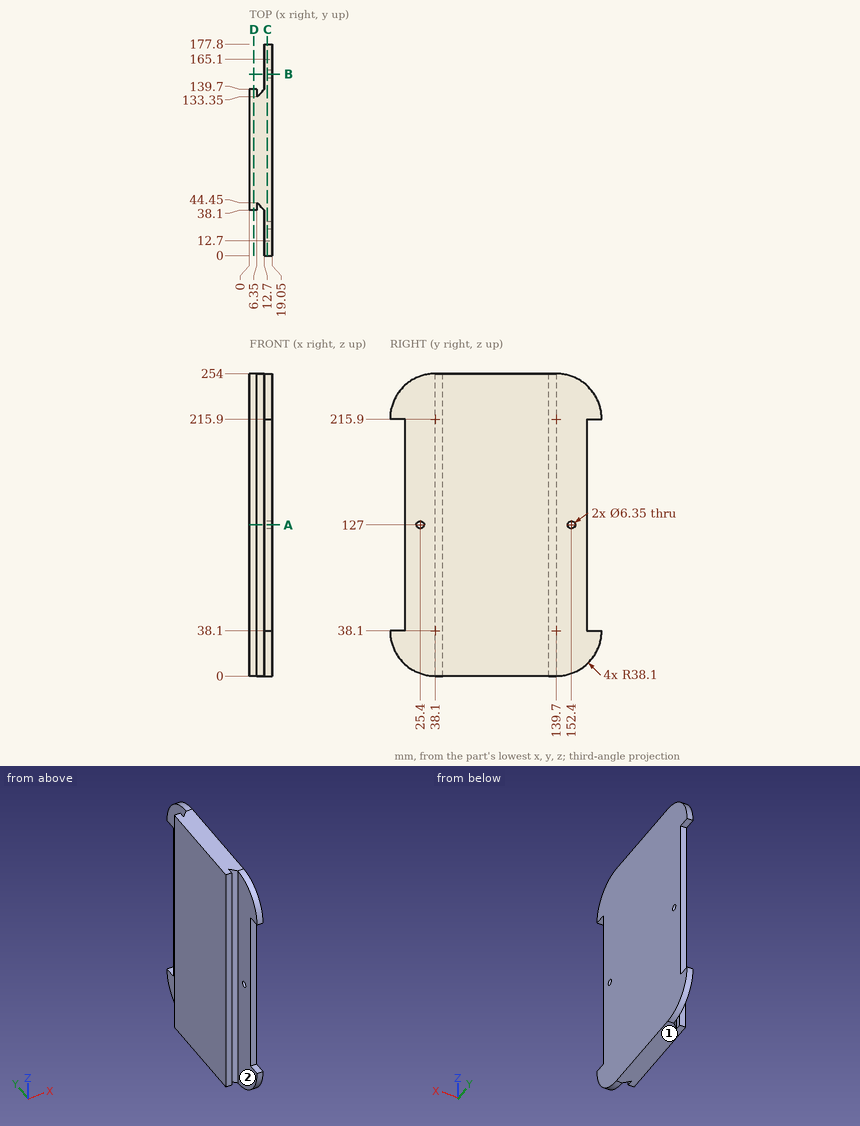
Here's the drawing with two shaded views (mm, measured from the low corner). I have some questions. A direction names the side the tool comes from. Round coordinates to 2 decimals unless told otherwise and drop trailing zeros. Loops run counter-clockwise (first coordinate to the right, second up) from the corner with the lowest first, then second, coordinate; pieces in that order, holes last.
Item 1: Suppose I cut it at C-C, the plane x = 15.25. Write out the boundary of the cut face in (y, z) (3 decimals).
Item 2: Suppose I cut it at B-B, the plane y = 152.4. Write out the boundary of the cut face in (x, z) (3 decimals), then the cut area to 3 significant figures.
Item 3: Suppose I cut it at D-D, the plane x = 3.75. Write out the boundary of the cut face in (y, z), then the cut area to 3 significant figures.
Item 4: Which directions (+Z, -Z, +X, -X, +Y, -Y) give clear straight access to the entire face, cutting with the end or side of a thin tool? Please do the marked faces 1 and 2.
Item 5: Suppose I cut it at A-A, the plane z = 127. Write out the boundary of the cut face in (x, y) (3 decimals).
Item 6: Will these pins go through, and if not, where does the flat tip stop? pin 1 Ø1.9 at (x, z) = (15.5, 133.5) entering from +Y; pin 2 Ø5 at (x, y) = (16.5, 174) entering from +Z (3 decimals); pin 3 Ø8.5 at (y, z) = (25.4, 127) entering from +X; pin 4 Ø3 at (x, z) = (1.5, 107) entering from -Y.
Item 7: Please list where these lines run through material, in increasing order: L1, parallel to Y at x = 14, z = 127 (3 decimals); L2, parallel to Y at x = 4.5, z = 175.5; L3, parallel to X at y = 150.5, z = 163.
Reported:
1. outline: (0, 38.1) arc R38.1 ccw to (38.1, 0) - (139.7, 0) arc R38.1 ccw to (177.8, 38.1) - (165.1, 38.1) - (165.1, 215.9) - (177.8, 215.9) arc R38.1 ccw to (139.7, 254) - (38.1, 254) arc R38.1 ccw to (0, 215.9) - (12.7, 215.9) - (12.7, 38.1) - close; hole circle Ø6.35 at (25.4, 127); hole circle Ø6.35 at (152.4, 127)
2. outline: (12.7, 2.179) - (19.05, 2.179) - (19.05, 123.825) - (12.7, 123.825) - close; (12.7, 130.175) - (19.05, 130.175) - (19.05, 251.821) - (12.7, 251.821) - close
2. area: 1,540 mm2
3. outline: (38.1, 0) - (139.7, 0) - (139.7, 254) - (38.1, 254) - close
3. area: 25,800 mm2
4. face 1: -Z, +X, -X, +Y, -Y
4. face 2: +Z, -Z, -X, -Y
5. outline: (0, 38.1) - (6.35, 38.1) - (6.35, 44.45) - (12.7, 38.1) - (12.7, 28.575) - (19.05, 28.575) - (19.05, 149.225) - (12.7, 149.225) - (12.7, 139.7) - (6.35, 133.35) - (6.35, 139.7) - (0, 139.7) - close; (12.7, 12.7) - (19.05, 12.7) - (19.05, 22.225) - (12.7, 22.225) - close; (12.7, 155.575) - (19.05, 155.575) - (19.05, 165.1) - (12.7, 165.1) - close
6. pin 1: stops at y = 165.1
6. pin 2: stops at z = 236.885
6. pin 3: stops at x = 19.05
6. pin 4: stops at y = 38.1
7. L1: y = 12.7 to 22.225, 28.575 to 149.225, 155.575 to 165.1
7. L2: y = 38.1 to 139.7
7. L3: x = 12.7 to 19.05
